Can you work these out from the model? Positions are in its coordinate system, mm. A direction names the side the tool comes from. Give positions to 0.01 mm unless a question says otherwise; leave off trailing zeros. Write each loop counter-clockwise with the first axis right and the second up, starting at its lowest first coordinate (ties: lowest second). Pieces come first, ordered by that corner, then holes.
```python
from build123d import *

# Parameters (mm, degrees)
BOSS_EXTRUDE1_DEPTH = 12.5
SKETCH3_R           = 1.5
CUT_EXTRUDE1_DEPTH  = 12.5
SKETCH4_W           = 3
SKETCH4_H           = 9.5
CUT_EXTRUDE2_DEPTH  = 5
SKETCH5_R           = 1
CUT_EXTRUDE3_DEPTH  = 3


with BuildPart() as part:
    # Sketch2 → Boss-Extrude1 (new body)
    with BuildSketch(Plane(origin=(0, 0, 0), x_dir=(0, 0, -1), z_dir=(1, 0, 0))):
        Polygon((6, 0), (25, 0), (25, 12.5), (48, 12.5), (48, 0), (61, 0), (61, -4.5), (67, -4.5), (67, 0), (67, 3), (53, 3), (53, 17.5), (20, 17.5), (20, 3), (0, 3), (0, 0), (0, -4.5), (6, -4.5), align=None)
    extrude(amount=BOSS_EXTRUDE1_DEPTH)

    # Sketch3 → Cut-Extrude1 (cut)
    with BuildSketch(Plane(origin=(0, 3, 0), x_dir=(1, 0, 0), z_dir=(0, 1, 0))):
        with Locations((7.5, 3)):
            Circle(SKETCH3_R)
        with Locations((7.5, 64)):
            Circle(SKETCH3_R)
    extrude(amount=-CUT_EXTRUDE1_DEPTH, mode=Mode.SUBTRACT)

    # Sketch4 → Cut-Extrude2 (cut)
    with BuildSketch(Plane.XY.offset(-20)):
        with Locations((1.5, 7.75)):
            Rectangle(SKETCH4_W, SKETCH4_H)
    extrude(amount=-CUT_EXTRUDE2_DEPTH, mode=Mode.SUBTRACT)

    # Sketch5 → Cut-Extrude3 (cut)
    with BuildSketch(Plane(origin=(12.5, 0, 0), x_dir=(0, 0, -1), z_dir=(1, 0, 0))):
        with Locations((22.65, 6.25)):
            Circle(SKETCH5_R)
        with Locations((50.35, 6.25)):
            Circle(SKETCH5_R)
    extrude(amount=-CUT_EXTRUDE3_DEPTH, mode=Mode.SUBTRACT)


solid = part.part
```
1) Suppose I cut it at C-C on y = 6.25. Write out the boundary of the cut face in (x, z), plus the area to 3 significant figures.
Values follow:
outline: (0, -53) - (12.5, -53) - (12.5, -51.35) - (9.5, -51.35) - (9.5, -49.35) - (12.5, -49.35) - (12.5, -48) - (0, -48) - close; (3, -25) - (12.5, -25) - (12.5, -23.65) - (9.5, -23.65) - (9.5, -21.65) - (12.5, -21.65) - (12.5, -20) - (3, -20) - close
area: 98.0 mm2
2) Suppose I cut it at D-D on z = -22.65. Write out the boundary of the cut face in (x, y), plus the area to 3 significant figures.
Values follow:
outline: (0, 0) - (12.5, 0) - (12.5, 5.25) - (9.5, 5.25) - (9.5, 7.25) - (12.5, 7.25) - (12.5, 17.5) - (0, 17.5) - (0, 12.5) - (3, 12.5) - (3, 3) - (0, 3) - close
area: 184 mm2
3) Please list where these lines run through material, in increasing order: L1, parallel to Z at x = 7.5, y = 0.5; L2, parallel to X at y = 1.25, z = -64; L3, parallel to Z at x = 3.75, y = -2.5.
Values follow:
L1: z = -67 to -65.5, -62.5 to -48, -25 to -4.5, -1.5 to 0
L2: x = 0 to 6, 9 to 12.5
L3: z = -67 to -61, -6 to 0
4) Suppose I cut it at A-A on y = 1. Write out the boundary of the cut face in (x, z), plus the area to 3 significant figures.
Values follow:
outline: (0, -67) - (12.5, -67) - (12.5, -48) - (0, -48) - close; (0, -25) - (12.5, -25) - (12.5, 0) - (0, 0) - close; hole circle Ø3 at (7.5, -64); hole circle Ø3 at (7.5, -3)
area: 536 mm2
5) For faces 1 (the face through (9.5, 6, -50)), 2 (the face through (3, 8, -22)), 3 (the face through (6, 6, -48)), 4 (the face through (6, -4.5, -2)), which set-ups out of +Z, -Z, +X, -X, +Y, -Y let a thin tool reach every point of the face, with its end or its side?
Values follow:
face 1: +X
face 2: +Z, -X
face 3: +X, -X, -Y
face 4: +Z, -Z, +X, -X, -Y
6) For pin 1 Ø6 at (x, z) = (7.5, -39.5) entering from -Y; pin 2 Ø1.8 at (y, z) = (6.25, -22.65) entering from -X; pin 3 Ø5 at (x, z) = (8, -11) entering from +Y; pin 4 Ø2.5 at (x, z) = (7.5, -3) entering from +Y, each with a flat end and sliding along its axis, tell me the tip position at first contact or that it passes through.
Values follow:
pin 1: stops at y = 12.5
pin 2: stops at x = 3
pin 3: stops at y = 3
pin 4: passes through
7) If we mould it in two halves opening along Z, with no side actions, what happens to faces 5 (the face through (0, 13, -45)), 6 (the face through (8, 10, -20)), 7 (the face through (6, -2, -61))? For each: +Z half, -Z half, draft (parallel to the pull), parting line (faces both ways), or undercut.
Values follow:
face 5: draft
face 6: +Z half
face 7: undercut
8) Suppose I cut it at B-B on x = 2.25. Write out the boundary of the cut face in (y, z), plus the area to 4 significant figures.
Values follow:
outline: (-4.5, -67) - (3, -67) - (3, -53) - (17.5, -53) - (17.5, -20) - (12.5, -20) - (12.5, -48) - (0, -48) - (0, -61) - (-4.5, -61) - close; (-4.5, -6) - (0, -6) - (0, -25) - (3, -25) - (3, 0) - (-4.5, 0) - close
area: 398.5 mm2
